```python
from build123d import *

# Parameters (mm, degrees)
SKETCH2_W           = 160
SKETCH2_H           = 15
BOSS_EXTRUDE1_DEPTH = 4
BOSS_EXTRUDE2_DEPTH = 4
SKETCH5_R           = 1.5
CUT_EXTRUDE1_DEPTH  = 82.229612827
CUT_EXTRUDE2_DEPTH  = 82.229612827
FILLET1_R           = 7
FILLET2_R           = 2
CUT_EXTRUDE3_DEPTH  = 82.229612947


with BuildPart() as part:
    # Sketch2 → Boss-Extrude1 (new body)
    with BuildSketch(Plane(origin=(0, 0, 0), x_dir=(1, 0, 0), z_dir=(0, 1, 0))):
        Rectangle(SKETCH2_W, SKETCH2_H)
    extrude(amount=BOSS_EXTRUDE1_DEPTH)

    # Sketch4 → Boss-Extrude2 (add)
    with BuildSketch(Plane(origin=(0, 0, 0), x_dir=(1, 0, 0), z_dir=(0, 1, 0))):
        with BuildLine():
            Line((-45, -7.5), (-33, -7.5))
            ThreePointArc((-33, -7.5), (-39, -13.5), (-45, -7.5))
        make_face()
    extrude(amount=BOSS_EXTRUDE2_DEPTH)

    # Sketch5 → Cut-Extrude1 (cut, through all)
    with BuildSketch(Plane(origin=(0, 4, 0), x_dir=(1, 0, 0), z_dir=(0, 1, 0))):
        with Locations(Location((-77, 0, 0), (0, 0, 270))):
            Circle(SKETCH5_R)
        with Locations(Location((-39, -9.5, 0), (0, 0, 270))):
            Circle(SKETCH5_R)
        with Locations(Location((77, -4.5, 0), (0, 0, 270))):
            Circle(SKETCH5_R)
    extrude(amount=-CUT_EXTRUDE1_DEPTH, mode=Mode.SUBTRACT)

    # Sketch6 → Cut-Extrude2 (cut, through all)
    with BuildSketch(Plane(origin=(0, 4, 0), x_dir=(1, 0, 0), z_dir=(0, 1, 0))):
        with BuildLine():
            Line((80, 7.5), (-8.231546833, 7.5))
            add(Edge.make_bspline(
                [(-8.231546833, 7.5), (14.290081903, 5.870335425), (49.538058278, 2.848640909), (69.508001123, -0.069415723), (80, -1.449425232)],
                knots=[0, 0, 0, 0, 0, 1, 1, 1, 1, 1], degree=4))
            Line((80, -1.449425232), (80, 7.5))
        make_face()
    extrude(amount=-CUT_EXTRUDE2_DEPTH, mode=Mode.SUBTRACT)

    # Fillet1
    fillet1_edges = [part.edges().sort_by_distance(p)[0] for p in [
        (-80, 2, -7.5),
        (-80, 2, 7.5),
    ]]
    fillet(fillet1_edges, radius=FILLET1_R)

    # Fillet2
    # the kernel refuses this fillet: 2 mm, written as the material it takes off along each edge
    with BuildSketch(Plane(origin=(-8.231546833, 4, -7.5), x_dir=(-1, 0, 0), z_dir=(0, -1, 0))) as fillet2_piece_1:
        with BuildLine():
            CenterArc((0.072290514, -2), FILLET2_R, 90, 4.141569808)
            Line((-0.072151683, -0.005222706), (-0.075040527, 0.03467284))
            ThreePointArc((-0.075040527, 0.03467284), (-0.038963722, 0.037284715), (-0.002886851, 0.03989569))
            Line((-0.002886851, 0.03989569), (0, 0.04))
            Line((0, 0.04), (0.072290514, 0.04))
            Line((0.072290514, 0.04), (0.072290514, 0))
        make_face()
    extrude(amount=4, mode=Mode.SUBTRACT)
    with BuildSketch(Plane(origin=(80, 0, 7.5), x_dir=(-1, 0, 0), z_dir=(0, 1, 0))) as fillet2_piece_2:
        with BuildLine():
            CenterArc((FILLET2_R, -FILLET2_R), FILLET2_R, 90, 90)
            Line((0, -FILLET2_R), (-FILLET2_R * 0.02, -FILLET2_R))
            Line((-FILLET2_R * 0.02, -FILLET2_R), (-FILLET2_R * 0.02, FILLET2_R * 0.02))
            Line((-FILLET2_R * 0.02, FILLET2_R * 0.02), (FILLET2_R, FILLET2_R * 0.02))
            Line((FILLET2_R, FILLET2_R * 0.02), (FILLET2_R, 0))
        make_face()
    extrude(amount=4, mode=Mode.SUBTRACT)
    with BuildSketch(Plane(origin=(80, 4, 1.449425232), x_dir=(-0.9912995401068606, 0, -0.13162530829565738), z_dir=(0, -1, 0))) as fillet2_piece_3:
        with BuildLine():
            CenterArc((1.751992616, -1.999999306), FILLET2_R, 90.047746208, 82.388731024)
            Line((-0.230606464, -1.736748689), (-0.270258446, -1.731483677))
            Line((-0.270258446, -1.731483677), (-0.039651982, 0.005265012))
            Line((-0.039651982, 0.005265012), (4.9175e-05, 0.03999997))
            ThreePointArc((4.9175e-05, 0.03999997), (0.875159086, 0.039555606), (1.750292626, 0.039999986))
            Line((1.750292626, 0.039999986), (1.750325959, 0))
        make_face()
    extrude(amount=4, mode=Mode.SUBTRACT)

    # Sketch7 → Cut-Extrude3 (cut, through all)
    with BuildSketch(Plane(origin=(0, 4, 0), x_dir=(1, 0, 0), z_dir=(0, 1, 0))):
        with BuildLine():
            Line((-73, -7.5), (-45, -7.5))
            ThreePointArc((-45, -7.5), (-59, -6.045404943), (-73, -7.5))
        make_face()
        with BuildLine():
            Line((-73, 7.5), (-45, 7.5))
            ThreePointArc((-45, 7.5), (-59, 6.045404943), (-73, 7.5))
        make_face()
    extrude(amount=-CUT_EXTRUDE3_DEPTH, mode=Mode.SUBTRACT)


solid = part.part
```
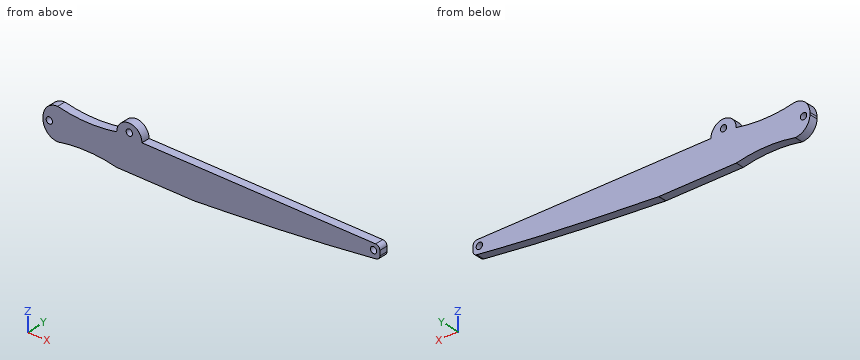
The model under review builds one solid part; all positions refer to its coordinate system, in mm. Round coordinates to 2 decimals unless told otherwise and drop trailing zeros. Loops run counter-clockwise (first coordinate to the right, second up) from the corner with the lowest first, then second, coordinate; pieces in that order, holes last.
1) Wall thickness on line 1 along Z through (x, y) = (-31, 0.3); line 2 along Z through (x, y) = (-77, 1.75); line 3 along X through (y, z) = (3.1, 4.5): over which ranges is each line inside the solid? List them lowest first.
Values follow:
line 1: z = -7.5 to 7.5
line 2: z = -6.24 to -1.5, 1.5 to 6.24
line 3: x = -78.74 to 75.5, 78.5 to 80
2) Consider section C-C on y = 1.75. Give the number of separate pieces and of enclosed holes in the cut face, then the cut area to 3 significant figures.
Values follow:
separate pieces: 1
enclosed holes: 3
area: 2,000 mm2
3) Clearance check with flat-ended pins moving along their axes: P1, Ø2, axis at y = 1.5, z = 2.5, coming from the -X side; P2, Ø1.2, axis at x = 8, y = 2.5, coming from the +Z side. State where each tip first meets the part, or that it passes through.
Values follow:
P1: stops at x = -79.93
P2: stops at z = 7.5
4) Consider section A-A on x = -39. State the section outline as (y, z) points.
Values follow:
outline: (0, -7.5) - (4, -7.5) - (4, 8) - (0, 8) - close; (0, 11) - (4, 11) - (4, 13.5) - (0, 13.5) - close
5) Consider section B-B on z = 9.5. State the section outline as (x, y) points.
Values follow:
outline: (-44.66, 0) - (-40.5, 0) - (-40.5, 4) - (-44.66, 4) - close; (-37.5, 0) - (-33.34, 0) - (-33.34, 4) - (-37.5, 4) - close
6) Consider section D-D on x = -59.5. State the section outline as (y, z) points, then the cut area to 3 significant figures.
Values follow:
outline: (0, -6.05) - (4, -6.05) - (4, 6.05) - (0, 6.05) - close
area: 48.4 mm2
